Autodesk Inventor part; units mm, degrees
ref_plane "YZ Plane" through (0, 0, 0) normal (1, 0, 0) x (0, 1, 0)
ref_plane "XZ Plane" through (0, 0, 0) normal (0, 1, 0) x (-1, 0, 0)
ref_plane "XY Plane" through (0, 0, 0) normal (0, 0, 1) x (1, 0, 0)
sketch "Sketch1" plane through (0, 0, 0) normal (0, 1, 0) x (-1, 0, 0)
  line L0 (10.136, 16.6006) -> (-75.904, 16.6006)
  line L1 (-75.904, 16.6006) -> (-75.904, -66.8994)
  line L2 (-75.904, -66.8994) -> (10.136, -66.8994)
  line L3 (10.136, -66.8994) -> (10.136, 16.6006)
  point P0 (0, 0)
  dimension "d0" = 86.04
  dimension "d1" = 83.5
extrude "Extrusion1" add sketch "Sketch1" along normal blind 2
sketch "Sketch2" plane through (0, 2, 0) normal (0, 1, 0) x (1, 0, 0)
  circle A0 centre (-5.136, -11.6006) radius 1.7
  line L0 (-10.136, 66.8994) -> (-10.136, -16.6006)
  line L1 (-10.136, -16.6006) -> (75.904, -16.6006)
  circle A1 centre (70.904, -11.6006) radius 1.7
  line L2 (75.904, -16.6006) -> (75.904, 66.8994)
  circle A2 centre (70.904, 61.8994) radius 1.7
  line L3 (75.904, 66.8994) -> (-10.136, 66.8994)
  circle A3 centre (-5.136, 61.8994) radius 1.7
  point P0 (0, 0)
  dimension "d4" = 3.4
  dimension "d5" = 5
  dimension "d6" = 5
  dimension "d7" = 3.4
  dimension "d8" = 5
  dimension "d9" = 5
  dimension "d10" = 3.4
  dimension "d11" = 5
  dimension "d12" = 5
  dimension "d13" = 3.4
  dimension "d14" = 5
  dimension "d15" = 5
extrude "Extrusion2" cut sketch "Sketch2" against normal blind 2 contours A0 | A1 | A2 | A3
sketch "Sketch3" plane through (0, 2, 0) normal (0, 1, 0) x (1, 0, 0)
  line L0 (6.834, -4.6006) -> (20.834, -4.6006)
  line L1 (20.834, -4.6006) -> (20.834, 9.3994)
  line L2 (20.834, 9.3994) -> (6.834, 9.3994)
  line L3 (6.834, 9.3994) -> (6.834, -4.6006)
  line L4 (25.884, 9.3994) -> (39.884, 9.3994)
  line L5 (39.884, 9.3994) -> (39.884, -4.6006)
  line L6 (39.884, -4.6006) -> (25.884, -4.6006)
  line L7 (25.884, -4.6006) -> (25.884, 9.3994)
  line L8 (44.934, 9.3994) -> (58.934, 9.3994)
  line L9 (58.934, 9.3994) -> (58.934, -4.6006)
  line L10 (58.934, -4.6006) -> (44.934, -4.6006)
  line L11 (44.934, -4.6006) -> (44.934, 9.3994)
  line L12 (6.834, 14.4494) -> (20.834, 14.4494)
  line L13 (20.834, 14.4494) -> (20.834, 28.4494)
  line L14 (20.834, 28.4494) -> (6.834, 28.4494)
  line L15 (6.834, 28.4494) -> (6.834, 14.4494)
  line L16 (25.884, 28.4494) -> (39.884, 28.4494)
  line L17 (39.884, 28.4494) -> (39.884, 14.4494)
  line L18 (39.884, 14.4494) -> (25.884, 14.4494)
  line L19 (25.884, 14.4494) -> (25.884, 28.4494)
  line L20 (44.934, 28.4494) -> (58.934, 28.4494)
  line L21 (58.934, 28.4494) -> (58.934, 14.4494)
  line L22 (58.934, 14.4494) -> (44.934, 14.4494)
  line L23 (44.934, 14.4494) -> (44.934, 28.4494)
  line L24 (-10.136, 66.8994) -> (-10.136, -16.6006)
  line L25 (-10.136, -16.6006) -> (75.904, -16.6006)
  line L26 (6.834, 35.5494) -> (45.834, 35.5494)
  line L27 (45.834, 35.5494) -> (45.834, 48.5494)
  line L28 (45.834, 48.5494) -> (6.834, 48.5494)
  line L29 (6.834, 48.5494) -> (6.834, 35.5494)
  circle A0 centre (53.834, 42.0494) radius 3.5
  point P0 (0, 0)
  point P1 (25.884, 21.4494)
  point P2 (20.834, 21.4494)
  point P3 (6.834, 21.4494)
  point P4 (32.884, 9.3994)
  point P5 (32.884, 14.4494)
  point P6 (32.884, -16.6006)
  point P7 (51.934, -4.6006)
  point P8 (13.834, 28.4494)
  point P9 (45.834, 42.0494)
  dimension "d18" = 14
  dimension "d19" = 14
  dimension "d20" = 14
  dimension "d21" = 5.05
  dimension "d22" = 14
  dimension "d23" = 5.05
  dimension "d24" = 14
  dimension "d25" = 14
  dimension "d26" = 5.05
  dimension "d27" = 14
  dimension "d28" = 14
  dimension "d29" = 14
  dimension "d30" = 14
  dimension "d31" = 5.05
  dimension "d32" = 5.05
  dimension "d33" = 5.05
  dimension "d34" = 16.97
  dimension "d35" = 5.05
  dimension "d39" = 12
  dimension "d40" = 12
  dimension "d41" = 12
  dimension "d42" = 39
  dimension "d43" = 13
  dimension "d44" = 7.1
  dimension "d45" = 7
  dimension "d46" = 8
extrude "Extrusion3" cut sketch "Sketch3" against normal blind 2
fillet "Fillet1" radius 5 4 edges at (-10.136, 1, 16.6006) (75.904, 1, 16.6006) (75.904, 1, -66.8994) (-10.136, 1, -66.8994)
properties part number "Case_Top"
Work out the finished part from the listing and answer in its coordinate system (mm). A direction names the side the tool comes from. Give positions to 0.01 mm unless a question says otherwise; leave off trailing zeros. Write each loop counter-clockwise with the first axis right and the second up, starting at its lowest first coordinate (ties: lowest second). Pieces come first, ordered by that corner, then holes. Notation, with made-up numbers: (-15.75, 16) - (23.25, 16) arc R15 ccw to (23.25, 37) - close; hole circle Ø9 at (-17, -31.5). An arc over 180 degrees is marked (long way). Use one line per item in the form item = value.
1. This flat-tipped pin is pushed along its axis until it touches: pin 1 Ø2.5 at (x, z) = (70.9, 11.6) entering from -Y. Where does it stop, or does it pass through?
Filled in:
pin_1 = through
2. Determine the mould class of faces 1 (the face through (33, 1, -66.899)), 2 (the face through (58.934, 1, -22)), 3 (the face through (74.478, 1.014, -65.396)) for opening direction X: released by +X, released by -X, zero draft, split by the parting line, or undercut.
Filled in:
face_1 = zero draft
face_2 = undercut
face_3 = released by +X
3. Consider L1, parallel to Z at x = 45, y = 0.55; L2, parallel to Z at x = 49, y = 1.2; L3, parallel to X at y = 0.45, z = -16. Determine where each line is inside the solid, lowest interval first.
Filled in:
L1 = -66.9 to -48.55, -35.55 to -28.45, -14.45 to -9.4, 4.6 to 16.6
L2 = -66.9 to -28.45, -14.45 to -9.4, 4.6 to 16.6
L3 = -10.14 to 6.83, 20.83 to 25.88, 39.88 to 44.93, 58.93 to 75.9
4. A cutting plane is placed at D-D (y = 1.35). State how many separate pieces and enclosed holes the cut face has, and give its area (3 significant figures).
Filled in:
separate_pieces = 1
enclosed_holes = 12
area = 5,410 mm^2
5. A cutting plane is placed at C-C (x = 11.5). Write down the section's boundary in (y, z), and give its area (3 significant figures).
Filled in:
outline = (0, -66.9) - (2, -66.9) - (2, -48.55) - (0, -48.55) - close; (0, -35.55) - (2, -35.55) - (2, -28.45) - (0, -28.45) - close; (0, -14.45) - (2, -14.45) - (2, -9.4) - (0, -9.4) - close; (0, 4.6) - (2, 4.6) - (2, 16.6) - (0, 16.6) - close
area = 85.0 mm^2
6. For faces 4 (the face through (-8.632, 1.014, -65.474)), 5 (the face through (14, 1, -28.449)), determine the directions among +Z, -Z, +X, -X, +Y, -Y from which every point of the face is accessible in a straight line to the end or side of a thin tool.
Filled in:
face_4 = -Z, -X, +Y, -Y
face_5 = +Y, -Y
7. A cutting plane is placed at A-A (z = -18.5). Write down the section's boundary in (x, y), and give its area (3 significant figures).
Filled in:
outline = (-10.14, 0) - (6.83, 0) - (6.83, 2) - (-10.14, 2) - close; (20.83, 0) - (25.88, 0) - (25.88, 2) - (20.83, 2) - close; (39.88, 0) - (44.93, 0) - (44.93, 2) - (39.88, 2) - close; (58.93, 0) - (75.9, 0) - (75.9, 2) - (58.93, 2) - close
area = 88.1 mm^2
8. A cutting plane is placed at B-B (x = 23). Write down the section's boundary in (y, z), and give its area (3 significant figures).
Filled in:
outline = (0, -66.9) - (2, -66.9) - (2, -48.55) - (0, -48.55) - close; (0, -35.55) - (2, -35.55) - (2, 16.6) - (0, 16.6) - close
area = 141 mm^2
